```python
from build123d import *

# Parameters (mm, degrees)
BOSS_EXTRUDE1_DEPTH     = 5
CUT_EXTRUDE1_DEPTH      = 24
CUT_EXTRUDE1_DEPTH_BACK = 24
SKETCH3_R               = 1.5
CUT_EXTRUDE2_DEPTH      = 91


with BuildPart() as part:
    # Sketch1 → Boss-Extrude1 (new body)
    with BuildSketch(Plane.XY):
        with BuildLine():
            Line((72.394590039, 19), (72.394590039, -19))
            ThreePointArc((72.394590039, -19), (68.394590039, -23), (64.394590039, -19))
            Line((64.394590039, -19), (64.394590039, 19))
            ThreePointArc((64.394590039, 19), (68.394590039, 23), (72.394590039, 19))
        make_face()
    extrude(amount=BOSS_EXTRUDE1_DEPTH)

    # Sketch2 → Cut-Extrude1 (cut, two sides)
    with BuildSketch(Plane(origin=(0, 0, 0), x_dir=(1, 0, 0), z_dir=(0, 1, 0))) as cut_extrude1_sk:
        Polygon((72.394590039, -5), (64.394590039, -2.088238126), (64.394590039, -5), align=None)
    extrude(amount=CUT_EXTRUDE1_DEPTH, mode=Mode.SUBTRACT)
    extrude(cut_extrude1_sk.sketch, amount=-CUT_EXTRUDE1_DEPTH_BACK, mode=Mode.SUBTRACT)

    # Sketch3 → Cut-Extrude2 (cut)
    with BuildSketch(Plane(origin=(6.86158929, 0, -18.852061635), x_dir=(0.939692621, 0, 0.342020143), z_dir=(-0.342020143, 0, 0.939692621))):
        with Locations((65.769891562, 19)):
            Circle(SKETCH3_R)
        with Locations((65.769891562, -19)):
            Circle(SKETCH3_R)
    extrude(amount=-CUT_EXTRUDE2_DEPTH, mode=Mode.SUBTRACT)


solid = part.part
```
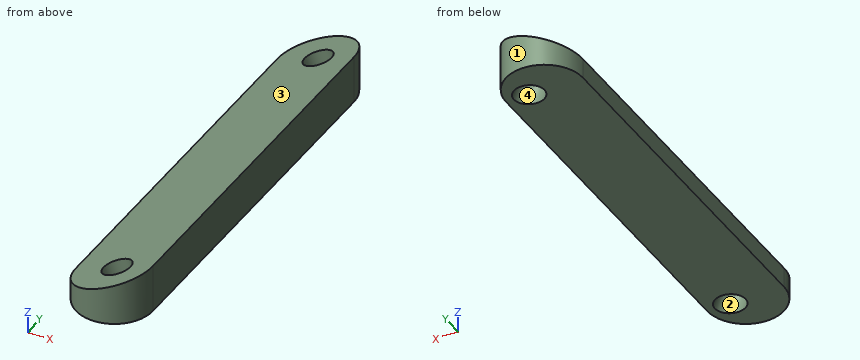
The model under review builds one solid part; all positions refer to its coordinate system, in mm. Face numbers are marked on the shaded views. Round coordinates to 2 decimals unless told otherwise and drop trailing zeros. Order: outer loops, then holes, each group sorted by start corner. A loop starts at its lowest first (then second) coordinate and runs counter-clockwise, first axis right, second up. Notation, with made-up numbers: M -27,40 L 26,40 A15 cw 26,56 Z; hole C 41.25,37.25 d6. An arc over 180 degrees is marked long. Use a Markdown table: item, result.
1) Insertion check: pin 1 (1.5 mm diameter, centred on x = 69.5, y = 15.5, fed in from +Z). The pin has a flat end and moves straight along its axis. Give the tip position at first contact, or say it passes through.
Report:
| item | result |
|---|---|
| pin 1 | z = 4.22 |
2) Consider section A-A (y = 5.5). Write out the cut boundary in (x, z), then the cut area to 3 significant figures.
Report:
| item | result |
|---|---|
| outline | M 64.39,0 L 72.39,0 L 72.39,5 L 64.39,2.09 Z |
| area | 28.4 mm^2 |
3) Consider section B-B (x = 69.25). Give the number of separate pieces and of enclosed holes in the cut face, then the cut area to 3 significant figures.
Report:
| item | result |
|---|---|
| separate pieces | 3 |
| enclosed holes | 0 |
| area | 154 mm^2 |
4) Draft analysis for pull direction Y (two halves, no side actions). For the marked faces 1, 2, 3 and 4, state which applies: released by +Y, released by -Y, zero draft, split by the parting line, or undercut.
Report:
| item | result |
|---|---|
| face 1 | released by +Y |
| face 2 | undercut |
| face 3 | zero draft |
| face 4 | undercut |
5) Wall thickness on line 1 along Y through (x, z) = (69.5, 3.8); line 2 along Y through (x, z) = (70, 1.15); line 3 along Y through (x, z) = (71.75, 2): over which ranges is each line inside the solid? List them lowest first. Write a range as [from, to].
Report:
| item | result |
|---|---|
| line 1 | [-22.84, -20.24], [-17.76, 17.76], [20.24, 22.84] |
| line 2 | [-22.66, -20.45], [-17.55, 17.55], [20.45, 22.66] |
| line 3 | [-21.18, 21.18] |
